from build123d import *

# Parameters (mm, degrees)
SKETCH1_W           = 100
SKETCH1_H           = 60
SKETCH1_R           = 1.5
BOSS_EXTRUDE1_DEPTH = 3
SKETCH3_R           = 1.5
SKETCH3_W           = 10
SKETCH3_H           = 17
BOSS_EXTRUDE2_DEPTH = 3
FILLET1_R           = 3
FILLET2_R           = 4


with BuildPart() as part:
    # Sketch1 → Boss-Extrude1 (new body)
    with BuildSketch(Plane(origin=(0, 0, 0), x_dir=(1, 0, 0), z_dir=(0, 1, 0))):
        Rectangle(SKETCH1_W, SKETCH1_H)
        with Locations((-29.462365137, -17.533964752)):
            Circle(SKETCH1_R, mode=Mode.SUBTRACT)
        with Locations((-29.462365137, -7.533964752)):
            Circle(SKETCH1_R, mode=Mode.SUBTRACT)
        with Locations((-29.462365137, 2.466035248)):
            Circle(SKETCH1_R, mode=Mode.SUBTRACT)
        with Locations((-29.462365137, 12.466035248)):
            Circle(SKETCH1_R, mode=Mode.SUBTRACT)
        with Locations((-29.462365137, 22.466035248)):
            Circle(SKETCH1_R, mode=Mode.SUBTRACT)
        with Locations((29.537634863, 22.466035248)):
            Circle(SKETCH1_R, mode=Mode.SUBTRACT)
        with Locations((29.537634863, 12.466035248)):
            Circle(SKETCH1_R, mode=Mode.SUBTRACT)
        with Locations((29.537634863, 2.466035248)):
            Circle(SKETCH1_R, mode=Mode.SUBTRACT)
        with Locations((29.537634863, -7.533964752)):
            Circle(SKETCH1_R, mode=Mode.SUBTRACT)
        with Locations((29.537634863, -17.533964752)):
            Circle(SKETCH1_R, mode=Mode.SUBTRACT)
    boss_extrude1 = extrude(amount=BOSS_EXTRUDE1_DEPTH)

    # Sketch3 → Boss-Extrude2 (add)
    with BuildSketch(Plane(origin=(50, 0, 0), x_dir=(0, 0, -1), z_dir=(1, 0, 0))):
        Polygon((-30, 3), (-25, 3), (-20, 3), (-20, 20), (-30, 20), align=None)
        with Locations((-25, 5.56)):
            Circle(SKETCH3_R, mode=Mode.SUBTRACT)
        with Locations((-25, 15.56)):
            Circle(SKETCH3_R, mode=Mode.SUBTRACT)
        with Locations((25, 11.5)):
            Rectangle(SKETCH3_W, SKETCH3_H)
        with Locations((25, 5.56)):
            Circle(SKETCH3_R, mode=Mode.SUBTRACT)
        with Locations((25, 15.56)):
            Circle(SKETCH3_R, mode=Mode.SUBTRACT)
    boss_extrude2 = extrude(amount=-BOSS_EXTRUDE2_DEPTH)

    # Mirror1: Boss-Extrude1, Boss-Extrude2 across plane
    add(boss_extrude1.mirror(Plane(origin=(0, 0, 0), x_dir=(0, 0, 1), z_dir=(1, 0, 0))))
    add(boss_extrude2.mirror(Plane(origin=(0, 0, 0), x_dir=(0, 0, 1), z_dir=(1, 0, 0))))

    # Fillet1
    fillet1_edges = [part.edges().sort_by_distance(p)[0] for p in [
        (48.5, 3, 20),
        (48.5, 3, -20),
        (-48.5, 3, 20),
        (-48.5, 3, -20),
    ]]
    fillet(fillet1_edges, radius=FILLET1_R)

    # Fillet2
    fillet2_edges = [part.edges().sort_by_distance(p)[0] for p in [
        (-48.5, 20, 30),
        (-48.5, 20, 20),
        (-48.5, 20, -20),
        (-48.5, 20, -30),
        (48.5, 20, -20),
        (48.5, 20, -30),
        (48.5, 20, 30),
        (48.5, 20, 20),
    ]]
    fillet(fillet2_edges, radius=FILLET2_R)


solid = part.part
Source: CAD feature listing. Evaluate the final solid. Frame: model axes, mm. A direction names the side the tool comes from. Round coordinates to 2 decimals unless told otherwise and drop trailing zeros. Order: outer loops, then holes, each group sorted by start corner. A loop starts at its lowest first (then second) coordinate and runs counter-clockwise, first axis right, second up. Notation, with made-up numbers: (-22.5, 50.5) -> (11.5, 50.5) arc R9 ccw to (11.5, 65.5) -> close; hole circle Ø1 at (-12, 68.25). An arc over 180 degrees is marked (long way). Answer as CSV lines item,"result".
Item 1: Reachability of faces 1 (the face through (-28.04, 1.48, -22.5)), 2 (the face through (-48.52, 14.65, 26.19)), 3 (the face through (-48.479, 18.859, -21.203)) from +Z, -Z, +X, -X, +Y, -Y: full face, straight path, thin tool, end or side. Return the list, or none.
A:
face 1,"+Y, -Y"
face 2,"+X, -X"
face 3,"+X, -X, +Y"
Item 2: Pin query (flat end, axial travel): pin 1 Ø12 at (x, z) = (-16.5, -18) entering from +Y. Return the tip coordinate at first contact, or that it passes through.
A:
pin 1,"y = 3"
Item 3: Pull-direction query (Z, two-part tool) for faces 4 (the face through (47, 12, -25)), 5 (the face through (10.9, 2.7, 30)), 6 (the face through (49, 11, 20)); classes: pulls with the +Z half, pulls with the -Z half, needs draft (parallel to the pull), parting line crosses it, or undercut.
A:
face 4,"needs draft"
face 5,"pulls with the +Z half"
face 6,"undercut"
Item 4: Section B-B, the plane y = 12. Return loops of the section in (x, z), plus the area to 3 significant figures.
A:
outline,"(-50, -30) -> (-47, -30) -> (-47, -20) -> (-50, -20) -> close; (-50, 20) -> (-47, 20) -> (-47, 30) -> (-50, 30) -> close; (47, -30) -> (50, -30) -> (50, -20) -> (47, -20) -> close; (47, 20) -> (50, 20) -> (50, 30) -> (47, 30) -> close"
area,"120 mm²"
Item 5: Section A-A, the plane z = -25. Return loops of the section in (x, y), plus the area to 3 significant figures.
A:
outline,"(-50, 0) -> (50, 0) -> (50, 4.06) -> (47, 4.06) -> (47, 3) -> (-47, 3) -> (-47, 4.06) -> (-50, 4.06) -> close; (-50, 7.06) -> (-47, 7.06) -> (-47, 14.06) -> (-50, 14.06) -> close; (-50, 17.06) -> (-47, 17.06) -> (-47, 20) -> (-50, 20) -> close; (47, 7.06) -> (50, 7.06) -> (50, 14.06) -> (47, 14.06) -> close; (47, 17.06) -> (50, 17.06) -> (50, 20) -> (47, 20) -> close"
area,"366 mm²"
Item 6: Line query: L1, parallel to Y at x = 49, z = 25; L2, parallel to X at y = 4.5, z = 27.5; L3, parallel to Y at x = 9, z = 20. Output: solid intervals per line, ascending.
A:
L1,"0 to 4.06, 7.06 to 14.06, 17.06 to 20"
L2,"-50 to -47, 47 to 50"
L3,"0 to 3"
Item 7: Section C-C, the plane x = -22. Return loops of the section in (y, z).
A:
outline,"(0, -30) -> (3, -30) -> (3, 30) -> (0, 30) -> close"
